from build123d import *

# Parameters (mm, degrees)
SKETCH1_W                                        = 101.6
SKETCH1_H                                        = 50.8
BOSS_EXTRUDE1_DEPTH                              = 25.4
CBORE_FOR_1_4_SOCKET_HEAD_CAP_SCREW1_D           = 6.7564
CBORE_FOR_1_4_SOCKET_HEAD_CAP_SCREW1_CBORE_D     = 11.1125
CBORE_FOR_1_4_SOCKET_HEAD_CAP_SCREW1_CBORE_DEPTH = 6.35
LPATTERN1_COUNT                                  = 2
LPATTERN1_PITCH                                  = 25.4
LPATTERN1_COUNT_DIR2                             = 4
LPATTERN1_PITCH_DIR2                             = 25.4
F_1_4_CLEARANCE_HOLE1_D                          = 6.7564
LPATTERN2_COUNT                                  = 4
LPATTERN2_PITCH                                  = 25.4
SKETCH7_W                                        = 101.6
SKETCH7_H                                        = 9.525
BOSS_EXTRUDE2_DEPTH                              = 19.05
LPATTERN3_COUNT                                  = 2
LPATTERN3_PITCH                                  = 25.4
LPATTERN4_COPY_1_D                               = 6.7564
LPATTERN4_COPY_2_D                               = 6.7564
SKETCH11_W                                       = 101.6
SKETCH11_H                                       = 9.525
BOSS_EXTRUDE3_DEPTH                              = 19.05
SKETCH8_W                                        = 50.8
SKETCH8_H                                        = 9.525
CUT_EXTRUDE1_DEPTH                               = 19.05
SKETCH12_W                                       = 50.8
SKETCH12_H                                       = 9.525
CUT_EXTRUDE2_DEPTH                               = 19.05
LPATTERN5_COUNT                                  = 2
LPATTERN5_PITCH                                  = 50.8
LPATTERN5_COUNT_DIR2                             = 2
LPATTERN5_PITCH_DIR2                             = 76.2


with BuildPart() as part:
    # Sketch1 → Boss-Extrude1 (new body)
    with BuildSketch(Plane(origin=(0, 0, 0), x_dir=(1, 0, 0), z_dir=(0, 1, 0))):
        with Locations((50.8, 25.4)):
            Rectangle(SKETCH1_W, SKETCH1_H)
    extrude(amount=BOSS_EXTRUDE1_DEPTH)

    # CBORE for 1/4 Socket Head Cap Screw1 (through all)
    with Locations(Plane(origin=(0, 25.4, 0), x_dir=(-1, 0, 0), z_dir=(0, 1, 0))):
        with Locations((-12.7, -12.7)):
            cbore_for_1_4_socket_head_cap_screw1 = CounterBoreHole(CBORE_FOR_1_4_SOCKET_HEAD_CAP_SCREW1_D / 2, CBORE_FOR_1_4_SOCKET_HEAD_CAP_SCREW1_CBORE_D / 2, CBORE_FOR_1_4_SOCKET_HEAD_CAP_SCREW1_CBORE_DEPTH)

    # LPattern1: CBORE for 1_4 Socket Head Cap Screw1 2 × 4
    with Locations(*[(j * LPATTERN1_PITCH_DIR2, 0, -i * LPATTERN1_PITCH) for i in range(LPATTERN1_COUNT) for j in range(LPATTERN1_COUNT_DIR2) if (i, j) != (0, 0)]):
        add(cbore_for_1_4_socket_head_cap_screw1, mode=Mode.SUBTRACT)

    # 1/4 Clearance Hole1 (through all)
    with Locations(Plane(origin=(0, 25.4, 0), x_dir=(-1, 0, 0), z_dir=(0, 1, 0))):
        with Locations((-12.7, -38.1)):
            f_1_4_clearance_hole1 = Hole(F_1_4_CLEARANCE_HOLE1_D / 2)

    # LPattern2: 1/4 Clearance Hole1 ×4
    with Locations(*[(-i * LPATTERN2_PITCH, 0, 0) for i in range(1, LPATTERN2_COUNT)]):
        add(f_1_4_clearance_hole1, mode=Mode.SUBTRACT)

    # Sketch7 → Boss-Extrude2 (add)
    with BuildSketch(Plane(origin=(0, 0, -50.8), x_dir=(-1, 0, 0), z_dir=(0, 0, -1))):
        with Locations((-50.8, 20.6375)):
            Rectangle(SKETCH7_W, SKETCH7_H)
    extrude(amount=BOSS_EXTRUDE2_DEPTH)

    # LPattern3: 1/4 Clearance Hole1 ×2
    with Locations(*[(0, 0, -i * LPATTERN3_PITCH) for i in range(1, LPATTERN3_COUNT)]):
        add(f_1_4_clearance_hole1, mode=Mode.SUBTRACT)

    # LPattern4 copy 1 (through all)
    with Locations(Plane(origin=(76.2, 25.4, -25.4), x_dir=(-1, 0, 0), z_dir=(0, 1, 0))):
        with Locations((-12.7, -38.1)):
            Hole(LPATTERN4_COPY_1_D / 2)

    # LPattern4 copy 2 (through all)
    with Locations(Plane(origin=(76.2, 25.4, 0), x_dir=(-1, 0, 0), z_dir=(0, 1, 0))):
        with Locations((-12.7, -38.1)):
            Hole(LPATTERN4_COPY_2_D / 2)

    # Sketch11 → Boss-Extrude3 (add)
    with BuildSketch(Plane.XY):
        with Locations((50.8, 20.6375)):
            Rectangle(SKETCH11_W, SKETCH11_H)
    extrude(amount=BOSS_EXTRUDE3_DEPTH)

    # Sketch8 → Cut-Extrude1 (cut)
    with BuildSketch(Plane(origin=(0, 0, -69.85), x_dir=(-1, 0, 0), z_dir=(0, 0, -1))):
        with Locations((-50.8, 20.6375)):
            Rectangle(SKETCH8_W, SKETCH8_H)
    extrude(amount=-CUT_EXTRUDE1_DEPTH, mode=Mode.SUBTRACT)

    # Sketch12 → Cut-Extrude2 (cut)
    with BuildSketch(Plane.XY.offset(19.05)):
        with Locations((50.8, 20.6375)):
            Rectangle(SKETCH12_W, SKETCH12_H)
    extrude(amount=-CUT_EXTRUDE2_DEPTH, mode=Mode.SUBTRACT)

    # LPattern5: 1_4 Clearance Hole1 2 × 2
    with Locations(*[(j * LPATTERN5_PITCH_DIR2, 0, i * LPATTERN5_PITCH) for i in range(LPATTERN5_COUNT) for j in range(LPATTERN5_COUNT_DIR2) if (i, j) != (0, 0)]):
        add(f_1_4_clearance_hole1, mode=Mode.SUBTRACT)


solid = part.part
Part model, mm, in its own coordinate system. A direction names the side the tool comes from. Round coordinates to 2 decimals unless told otherwise and drop trailing zeros. Order: outer loops, then holes, each group sorted by start corner. A loop starts at its lowest first (then second) coordinate and runs counter-clockwise, first axis right, second up. Notation, with made-up numbers: (-1.5, 73.5) -> (44.5, 73.5) arc R18 cw to (44.5, 94.5) -> close; hole circle Ø7 at (78.5, 7). An arc over 180 degrees is marked (long way). Put each result on its own line as item: value.
Q1. Band-saw the part on B-B (x = 88.9). State how many separate pieces and enclosed holes the cut face has, and give its area (3 significant figures).
From the geometry:
separate pieces: 5
enclosed holes: 0
area: 1,130 mm2
Q2. Band-saw the part on A-A (z = -52.5). Give the cut face in (x, y) (3 decimals).
From the geometry:
outline: (0, 15.875) -> (25.4, 15.875) -> (25.4, 25.4) -> (0, 25.4) -> close; (76.2, 15.875) -> (101.6, 15.875) -> (101.6, 25.4) -> (76.2, 25.4) -> close
Q3. Band-saw the part on C-C (x = 63.5). Give the cut face in (y, z).
From the geometry:
outline: (0, -50.8) -> (25.4, -50.8) -> (25.4, -43.66) -> (19.05, -43.66) -> (19.05, -41.48) -> (0, -41.48) -> close; (0, -34.72) -> (19.05, -34.72) -> (19.05, -32.54) -> (25.4, -32.54) -> (25.4, -18.26) -> (19.05, -18.26) -> (19.05, -16.08) -> (0, -16.08) -> close; (0, -9.32) -> (19.05, -9.32) -> (19.05, -7.14) -> (25.4, -7.14) -> (25.4, 0) -> (0, 0) -> close
Q4. Pin check, flat tips, straight feed: pin 1 Ø9 at (x, z) = (66, -40) entering from +Y; pin 2 Ø3 at (x, y) = (74.5, 15.5) entering from +Z; pin 3 Ø3 at (x, y) = (35, 10) entering from -Z; pin 4 Ø6 at (x, z) = (81.5, 4) entering from -Y (3 decimals). Stop position of each tip, or through.
From the geometry:
pin 1: stops at y = 25.4
pin 2: stops at z = 0
pin 3: stops at z = -50.8
pin 4: stops at y = 15.875
Q5. Tool access for faces 3 (the face through (89, 19.05, -16.3)), 4 (the face through (13, 15.875, -58)), 5 (the face through (76.2, 21, -60)), 6 (the face through (76.2, 21, 10)): list every direction of +Z, -Z, +X, -X, +Y, -Y with a clear straight run to the whole face (end or side of a thin tool).
From the geometry:
face 3: +Y
face 4: -Z, +X, -X, -Y
face 5: -Z, +Y, -Y
face 6: +Z, +Y, -Y
Q6. Wall check: line 1 (Z direction, x = 38.1, y = 9); line 2 (Z direction, x = 88.9, y = 18.75); line 3 (Z direction, x = 12.7, y = 22). Give the ranges that are in metal, low to high. Write a range as [from, to].
From the geometry:
line 1: z = [-50.8, -41.48], [-34.72, -16.08], [-9.32, 0]
line 2: z = [-69.85, -66.88], [-60.12, -41.48], [-34.72, -16.08], [-9.32, 9.32], [16.08, 19.05]
line 3: z = [-69.85, -66.88], [-60.12, -43.66], [-32.54, -18.26], [-7.14, 9.32], [16.08, 19.05]
Q7. Pull direction X, two halves, no side cores. Call faces 1 (the face through (89, 15.875, 7)), 2 (the face through (85.525, 20.571, 12.849)): pulls with the +X half, pulls with the -X half, needs draft (parallel to the pull), parting line crosses it, or undercut.
From the geometry:
face 1: needs draft
face 2: undercut
